Design review of the part built by this model. Coordinates are the model's own, in mm. A direction names the side the tool comes from. Give positions to 0.01 mm unless a question says otherwise; leave off trailing zeros. Write each loop counter-clockwise with the first axis right and the second up, starting at its lowest first coordinate (ties: lowest second). Pieces come first, ordered by that corner, then holes. Notation, with made-up numbers: M 23,40.5 L 81,40.5 A27 ccw 81,69.5 Z; hole C 5,79 d6. An arc over 180 degrees is marked long. Use a Markdown table: item, result. Add a question column.
```python
from build123d import *

# Parameters (mm, degrees)
BOSS_EXTRUDE1_DEPTH        = 10
CUT_EXTRUDE1_DEPTH         = 5
F_3_2_3_2_DIAMETER_HOLE1_D = 3.2
FILLET1_R                  = 2
CUT_EXTRUDE2_START         = -2.5
CUT_EXTRUDE2_DEPTH         = 2.5


with BuildPart() as part:
    # Sketch1 → Boss-Extrude1 (new body)
    with BuildSketch(Plane(origin=(0, 0, 0), x_dir=(1, 0, 0), z_dir=(0, 1, 0))):
        with BuildLine():
            ThreePointArc((-207.414551525, 32.851237658), (-210, 0), (-207.414551525, -32.851237658))
            Line((-207.414551525, -32.851237658), (-217.291434931, -34.415582309))
            ThreePointArc((-217.291434931, -34.415582309), (-220, 0), (-217.291434931, 34.415582309))
            Line((-217.291434931, 34.415582309), (-207.414551525, 32.851237658))
        make_face()
        with BuildLine():
            ThreePointArc((-217.291434931, -34.415582309), (-220, 0), (-217.291434931, 34.415582309))
            Line((-217.291434931, 34.415582309), (-220.254499953, 34.884885704))
            ThreePointArc((-220.254499953, 34.884885704), (-223, 0), (-220.254499953, -34.884885704))
            Line((-220.254499953, -34.884885704), (-217.291434931, -34.415582309))
        make_face()
        with BuildLine():
            Line((-204.451486503, 32.381934263), (-207.414551525, 32.851237658))
            ThreePointArc((-207.414551525, 32.851237658), (-210, 0), (-207.414551525, -32.851237658))
            Line((-207.414551525, -32.851237658), (-204.451486503, -32.381934263))
            ThreePointArc((-204.451486503, -32.381934263), (-207, 0), (-204.451486503, 32.381934263))
        make_face()
    extrude(amount=BOSS_EXTRUDE1_DEPTH)

    # Sketch15 → Cut-Extrude1 (cut)
    with BuildSketch(Plane(origin=(0, 10, 0), x_dir=(1, 0, 0), z_dir=(0, 1, 0))):
        with BuildLine():
            Line((-219.772609758, 10), (-209.761769634, 10))
            ThreePointArc((-209.761769634, 10), (-208.900850883, 21.457737542), (-207.414551525, 32.851237658))
            Line((-207.414551525, 32.851237658), (-217.291434931, 34.415582309))
            ThreePointArc((-217.291434931, 34.415582309), (-218.872736893, 22.242415451), (-219.772609758, 10))
        make_face()
        with BuildLine():
            ThreePointArc((-207.414551525, -32.851237658), (-208.900850883, -21.457737542), (-209.761769634, -10))
            Line((-209.761769634, -10), (-219.772609758, -10))
            ThreePointArc((-219.772609758, -10), (-218.872736893, -22.242415451), (-217.291434931, -34.415582309))
            Line((-217.291434931, -34.415582309), (-207.414551525, -32.851237658))
        make_face()
    extrude(amount=-CUT_EXTRUDE1_DEPTH, mode=Mode.SUBTRACT)

    # Ø3.2 (3.2) Diameter Hole1 (through all)
    with Locations(Plane(origin=(0, 0, 0), x_dir=(-1, 0, 0), z_dir=(0, -1, 0))):
        with Locations((214.18186009, -18.738484691), (214.18186009, 18.738484691)):
            Hole(F_3_2_3_2_DIAMETER_HOLE1_D / 2)

    # Fillet1
    fillet1_edges = [part.edges().sort_by_distance(p)[0] for p in [
        (-220.254499953, 5, 34.884885704),
        (-220.254499953, 5, -34.884885704),
        (-204.451486503, 5, -32.381934263),
        (-204.451486503, 5, 32.381934263),
    ]]
    fillet(fillet1_edges, radius=FILLET1_R)

    # Sketch19 → Cut-Extrude2 (cut)
    with BuildSketch(Plane.XZ.offset(CUT_EXTRUDE2_START)):
        with BuildLine():
            Line((-218.270184732, -34.570601048), (-206.417411405, -32.693306179))
            ThreePointArc((-206.417411405, -32.693306179), (-205.117889671, -31.901228423), (-204.75200014, -30.423978019))
            ThreePointArc((-204.75200014, -30.423978019), (-207, 0), (-204.75200014, 30.423978019))
            ThreePointArc((-204.75200014, 30.423978019), (-205.117889671, 31.901228423), (-206.417411405, 32.693306179))
            Line((-206.417411405, 32.693306179), (-218.270184732, 34.570601048))
            ThreePointArc((-218.270184732, 34.570601048), (-219.765933628, 34.207922413), (-220.561180845, 32.890203773))
            ThreePointArc((-220.561180845, 32.890203773), (-223, 0), (-220.561180845, -32.890203773))
            ThreePointArc((-220.561180845, -32.890203773), (-219.765933628, -34.207922413), (-218.270184732, -34.570601048))
        make_face()
    extrude(amount=CUT_EXTRUDE2_DEPTH, mode=Mode.SUBTRACT)


solid = part.part
```
(1) The part is to be moulded in two halves that separate along X. For faces 5 (the flat face through (-214, 2.5, 0)), 6 (the cylindrical face through (-205.13, 6.3, 31.92)), 7 (the cylindrical face through (-215.45, 3.77, -17.76)), say which applies: released by +X, released by -X, zero draft, split by the parting line, or undercut.
(2) Add section C-C on z = -12. Give the boundary of the cut face in (x, y).
(3) For pin 1 (3.5 mm diameter, centred on x = -216, z = 21, fed in from +Y); pin 2 (4 mm diameter, centred on y = 8, z = -11.5, fed in from -X); pin 3 (1.5 mm diameter, centred on x = -216, y = 3.5, fed in from +Z), all flat-tipped, find the tip position at first contact; note any pin that passes through.
(4) Machinability: for faces 1 (the cylindrical face through (-218.855, 7.535, -22.413)), 2 (the cylindrical face through (-208.884, 7.535, 21.618)), 3 (the cylindrical face through (-208.917, 7.535, -21.298)), 4 (the flat face through (-214, 10, 0)), which of the approach directions +Z, -Z, +X, -X, +Y, -Y give a long, thin tool a straight path to every point of the face, cutting with its end or side? Answer none if there is none.
(5) Add section B-B on x = -213.75. Give the boundary of the cut face in (y, z).
(6) Add section D-D on x = -208.5. Give the boundary of the cut face in (y, z), then the cut area to 3 significant figures.
(7) Add section A-A on y = 6.5. Give the boundary of the cut face in (x, z), then the cut area to 3 significant figures.
(8) Wall thickness on L1, parallel to Z at x = -214.75, y = 3.25; L2, parallel to Z at x = -214.5, y = 9; L3, parallel to Y at x = -213.25, z = -26: over which ranges is each line inside the solid? List them lowest first.
From the geometry:
| question | item | result |
|---|---|---|
| 1 | face 5 | zero draft |
| 1 | face 6 | released by +X |
| 1 | face 7 | undercut |
| 2 | outline | M -222.68,2.5 L -206.65,2.5 L -206.65,10 L -209.66,10 L -209.66,5 L -219.67,5 L -219.67,10 L -222.68,10 Z |
| 3 | pin 1 | stops at y = 5 |
| 3 | pin 2 | stops at x = -222.8 |
| 3 | pin 3 | stops at z = 34.33 |
| 4 | face 1 | +Y |
| 4 | face 2 | +Z, +Y |
| 4 | face 3 | -Z, +Y |
| 4 | face 4 | +Z, -Z, +X, -X, +Y |
| 5 | outline | M 2.5,-33.85 L 5,-33.85 L 5,-20.28 L 2.5,-20.28 Z; M 2.5,-17.2 L 5,-17.2 L 5,-10 L 10,-10 L 10,10 L 5,10 L 5,17.2 L 2.5,17.2 Z; M 2.5,20.28 L 5,20.28 L 5,33.85 L 2.5,33.85 Z |
| 6 | outline | M 2.5,-33.02 L 5,-33.02 L 5,-25.05 L 10,-25.05 L 10,25.05 L 5,25.05 L 5,33.02 L 2.5,33.02 Z |
| 6 | area | 416 mm^2 |
| 7 | outline | M -220.56,-32.89 A2 ccw -218.27,-34.57 L -217.29,-34.42 A220 cw -219.77,-10 L -209.76,-10 A210 ccw -207.41,-32.85 L -206.42,-32.69 A2 ccw -204.75,-30.42 A207 cw -204.75,30.42 A2 ccw -206.42,32.69 L -207.41,32.85 A210 ccw -209.76,10 L -219.77,10 A220 cw -217.29,34.42 L -218.27,34.57 A2 ccw -220.56,32.89 A223 ccw Z |
| 7 | area | 602 mm^2 |
| 8 | L1 | z = -34.01 to -20.23, -17.24 to 17.24, 20.23 to 34.01 |
| 8 | L2 | z = -10 to 10 |
| 8 | L3 | y = 2.5 to 5 |
